CAD build for the part. Positions are in the model's coordinates, mm. Coordinates: 2 decimals unless noted, no trailing zeros. Write each loop counter-clockwise with the first axis right and the second up, starting at its lowest first coordinate (ties: lowest second). Pieces come first, ordered by that corner, then holes. Notation, with made-up numbers: M -17,27 L 37,27 A25 cw 37,54 Z; hole C -31,-36 d3. An arc over 180 degrees is marked long. Put each result on its own line as item: value. Start each with the question number.
```python
from build123d import *

# Parameters (mm, degrees)
SKETCH1_W           = 196.85
SKETCH1_H           = 107.95
BOSS_EXTRUDE1_DEPTH = 6.35
SKETCH2_W           = 57.15
SKETCH2_H           = 6.35
SKETCH2_W_2         = 6.35
SKETCH2_H_2         = 82.55
CUT_EXTRUDE1_DEPTH  = 154.060029074


with BuildPart() as part:
    # Sketch1 → Boss-Extrude1 (new body)
    with BuildSketch(Plane.XY):
        with Locations((-15.875, 47.625)):
            Rectangle(SKETCH1_W, SKETCH1_H)
    extrude(amount=-BOSS_EXTRUDE1_DEPTH)

    # Sketch2 → Cut-Extrude1 (cut, through all)
    with BuildSketch(Plane.XY):
        with BuildLine():
            Line((0, 101.6), (0, 95.25))
            ThreePointArc((0, 95.25), (-7.439487758, 77.289487758), (-25.4, 69.85))
            Line((-25.4, 69.85), (-25.4, 63.5))
            Line((-25.4, 63.5), (-107.95, 63.5))
            Line((-107.95, 63.5), (-107.95, 57.15))
            Line((-107.95, 57.15), (-114.3, 57.15))
            Line((-114.3, 57.15), (-114.3, 69.85))
            Line((-114.3, 69.85), (-114.3, 101.6))
            Line((-114.3, 101.6), (0, 101.6))
        make_face()
        with Locations((41.275, 98.425)):
            Rectangle(SKETCH2_W, SKETCH2_H)
        with Locations((79.375, 47.625)):
            Rectangle(SKETCH2_W_2, SKETCH2_H_2)
        Polygon((-114.3, -6.35), (-101.6, -6.35), (-101.6, 0), (-107.95, 0), (-107.95, 6.35), (-114.3, 6.35), align=None)
        with Locations((73.025, -3.175)):
            Rectangle(SKETCH2_W_2, SKETCH2_H)
    extrude(amount=-CUT_EXTRUDE1_DEPTH, mode=Mode.SUBTRACT)


solid = part.part
```
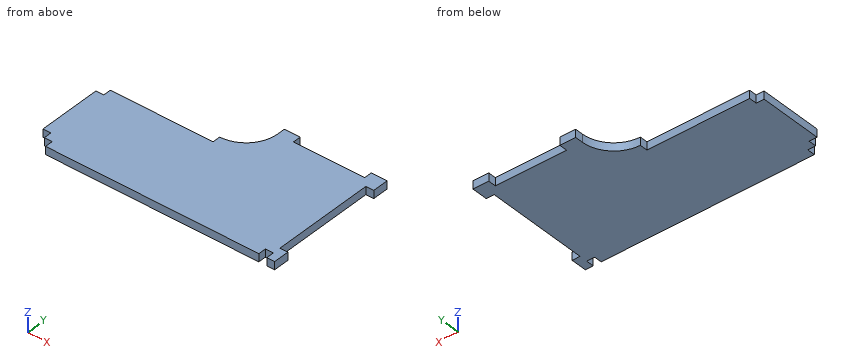
(1) Slice it at C-C, the plane y = 13. Write the cut outline in (x, z), then the cut area to 3 significant figures.
(2) Slice it at A-A, the plane z = -3. Write the cut outline in (x, y).
(3) Slice it at B-B, the plane x = 50. Write the cut outline in (y, z), then the cut area to 3 significant figures.
(4) Drill centre lines: line 1 (X direction, y = 96, z = -2.25); line 2 (X direction, y = 40, z = -5.5); line 3 (Y direction, x = -52.5, z = -3.5). Where is each one in solid material? Low to high. Write a range as [from, to].
(5) Drop flat-ended pins along their axis: pin 1 (1.9 mm diameter, centred on y = 98.5, z = -3, fed in from -X); pin 2 (3 mm diameter, centred on y = 42, z = -1.5, fed in from +X); pin 3 (1.9 mm diameter, centred on x = -84.5, z = -2.5, fed in from +Y); pin 4 (5 mm diameter, centred on x = -89, y = 44.5, fed in from +Z). Give the stop position or say it passes through.
Result set:
1. outline: M -114.3,-6.35 L 76.2,-6.35 L 76.2,0 L -114.3,0 Z
1. area: 1,210 mm^2
2. outline: M -114.3,6.35 L -107.95,6.35 L -107.95,0 L -101.6,0 L -101.6,-6.35 L 69.85,-6.35 L 69.85,0 L 76.2,0 L 76.2,-6.35 L 82.55,-6.35 L 82.55,6.35 L 76.2,6.35 L 76.2,88.9 L 82.55,88.9 L 82.55,101.6 L 69.85,101.6 L 69.85,95.25 L 12.7,95.25 L 12.7,101.6 L 0,101.6 L 0,95.25 A25.4 cw -25.4,69.85 L -25.4,63.5 L -107.95,63.5 L -107.95,57.15 L -114.3,57.15 Z
3. outline: M -6.35,-6.35 L 95.25,-6.35 L 95.25,0 L -6.35,0 Z
3. area: 645 mm^2
4. line 1: x = [0, 12.7], [69.85, 82.55]
4. line 2: x = [-114.3, 76.2]
4. line 3: y = [-6.35, 63.5]
5. pin 1: stops at x = 0
5. pin 2: stops at x = 76.2
5. pin 3: stops at y = 63.5
5. pin 4: stops at z = 0
